Geometry check sheet. Reference: the model listing, model coordinates, mm. Face numbers are marked on the shaded views. A direction names the side the tool comes from. Give positions to 0.01 mm unless a question says otherwise; leave off trailing zeros. Loops run counter-clockwise (first coordinate to the right, second up) from the corner with the lowest first, then second, coordinate; pieces in that order, holes last.
```python
from build123d import *

# Parameters (mm, degrees)
SIDE_BASE_DEPTH                    = 0.5
SIDE_BASE_2_COUNT                  = 2
SIDE_BASE_2_PITCH                  = 50
FRONT_BACK_WALLS_REACH             = 60.566
BASE_SKETCH_W                      = 50.5
BASE_SKETCH_H                      = 13.2
BASE_SKETCH_W_2                    = 15.8
BASE_SKETCH_H_2                    = 11.998021326
BASE_DEPTH                         = 0.5
ATTACHMENT_BASE_SKETCH_W           = 16.8
ATTACHMENT_BASE_SKETCH_H           = 13.2
ATTACHMENT_BASE_SKETCH_W_2         = 15.8
ATTACHMENT_BASE_SKETCH_H_2         = 11.998021326
ATTACHMENT_BASE_DEPTH              = 7
PIPE_TOP_EXTRA_CUTAWAY_REACH       = 64.84
SKETCH11_W                         = 15.8
SKETCH11_H                         = 0.195081796
SKETCH1_W                          = 15.8
SKETCH1_H                          = 12.193103122
FAN_BASE_DEPTH                     = 0.1
LEFT_RIGHT_WALL_REMOVAL_DEPTH      = 59.566323483
LEFT_RIGHT_WALL_REMOVAL_DEPTH_BACK = 59.566323483
SKETCH6_W                          = 28.631700026
SKETCH6_H                          = 16.366666667
CUTAWAY_LEFT_DEPTH                 = 53.811785181
LEFT_WALL_DEPTH                    = 0.520740187
SKETCH9_W                          = 43.808738797
SKETCH9_H                          = 16.366666667
CUTAWAY_RIGHT_DEPTH                = 46.956653807
RIGHT_WALL_DEPTH                   = 0.781709206


with BuildPart() as part:
    # Side base sketch → Side base (new body)
    with BuildSketch(Plane.ZY):
        Polygon((0, 13.2), (8.491348573, 5), (19.491348573, 0.8030407), (27.491348573, -0.530292633), (19, -3.166666667), (6, -1), (0, 0), align=None)
    extrude(amount=-SIDE_BASE_DEPTH)


with BuildPart() as side_base_2_1:
    # Side base 2: pattern copy
    add(part.part.moved(Location(Vector(1, 0, 0) * (1 * SIDE_BASE_2_PITCH))))

    # Wall base sketch → Front back walls (add, up to next)
    with BuildSketch(Plane(origin=(0.5, 0, 0), x_dir=(0, 0, -1), z_dir=(1, 0, 0)), mode=Mode.PRIVATE) as front_back_walls_sk1:
        Polygon((0, 12.504918204), (-8.217574488, 4.569298766), (-19.359827502, 0.318064001), (-26.428993119, -0.860130268), (-27.491348573, -0.530292633), (-19.491348573, 0.8030407), (-8.491348573, 5), (0, 13.2), align=None)
    front_back_walls_tool1 = extrude(front_back_walls_sk1.sketch, amount=FRONT_BACK_WALLS_REACH, mode=Mode.PRIVATE) - side_base_2_1.part
    # Wall base sketch → Front back walls (add, up to next)
    with BuildSketch(Plane(origin=(0.5, 0, 0), x_dir=(0, 0, -1), z_dir=(1, 0, 0)), mode=Mode.PRIVATE) as front_back_walls_sk2:
        Polygon((0, 0.506896878), (-19, -2.659769789), (-19, -3.166666667), (0, 0), align=None)
    front_back_walls_tool2 = extrude(front_back_walls_sk2.sketch, amount=FRONT_BACK_WALLS_REACH, mode=Mode.PRIVATE) - side_base_2_1.part

    add(part.part)  # Front back walls merges part
    add(front_back_walls_tool1.solids().sort_by_distance((0.5, 8.759227, 4.323285))[0])
    add(front_back_walls_tool2.solids().sort_by_distance((0.5, -1.329885, 9.5))[0])

    # Base sketch → Base (add)
    with BuildSketch(Plane(origin=(0, 0, 0), x_dir=(-1, 0, 0), z_dir=(0, 0, -1))):
        with Locations((-25.25, 6.6)):
            Rectangle(BASE_SKETCH_W, BASE_SKETCH_H)
        with Locations((-42.1, 6.505907541)):
            Rectangle(BASE_SKETCH_W_2, BASE_SKETCH_H_2, mode=Mode.SUBTRACT)
    extrude(amount=BASE_DEPTH)

    # Attachment base sketch → Attachment base (add)
    with BuildSketch(Plane(origin=(0, 0, -0.5), x_dir=(-1, 0, 0), z_dir=(0, 0, -1))):
        with Locations((-42.1, 6.6)):
            Rectangle(ATTACHMENT_BASE_SKETCH_W, ATTACHMENT_BASE_SKETCH_H)
        with Locations((-42.1, 6.505907541)):
            Rectangle(ATTACHMENT_BASE_SKETCH_W_2, ATTACHMENT_BASE_SKETCH_H_2, mode=Mode.SUBTRACT)
    extrude(amount=ATTACHMENT_BASE_DEPTH)

    # Pipe top extra cutaway: up to this plane
    pipe_top_extra_cutaway_end = Plane(origin=(500000, 12.504918204, 0), z_dir=(0, 0.7193398003386524, 0.694658370458996))
    # Sketch11 → Pipe top extra cutaway (cut, up to the surface)
    with BuildSketch(Plane(origin=(0, 0, -7.5), x_dir=(-1, 0, 0), z_dir=(0, 0, -1)), mode=Mode.PRIVATE) as pipe_top_extra_cutaway_sk1:
        with Locations((-42.1, 12.602459102)):
            Rectangle(SKETCH11_W, SKETCH11_H)
    pipe_top_extra_cutaway_tool1 = split(extrude(pipe_top_extra_cutaway_sk1.sketch, amount=-PIPE_TOP_EXTRA_CUTAWAY_REACH, mode=Mode.PRIVATE), bisect_by=pipe_top_extra_cutaway_end, keep=Keep.BOTH, mode=Mode.PRIVATE)
    add(pipe_top_extra_cutaway_tool1.solids().sort_by_distance((42.1, 12.602459, -7.5))[0], mode=Mode.SUBTRACT)

    # Sketch4 → Left right wall removal (cut, two sides: drawn at the far end of the back side and taken through both)
    with BuildSketch(Plane(origin=(0.5, 0, 0), x_dir=(0, 0, -1), z_dir=(1, 0, 0)).offset(-LEFT_RIGHT_WALL_REMOVAL_DEPTH_BACK)):
        Polygon((-26.428993119, -0.860130268), (-19, -3.166666667), (-19, -2.659769789), (0, 0.506896878), (0, 12.504918204), (-8.217574488, 4.569298766), (-19.359827502, 0.318064001), align=None)
    extrude(amount=LEFT_RIGHT_WALL_REMOVAL_DEPTH + LEFT_RIGHT_WALL_REMOVAL_DEPTH_BACK, mode=Mode.SUBTRACT)

    # Sketch6 → Cutaway left (cut, through all)
    with BuildSketch(Plane(origin=(46.557451165, 0, 13.548248036), x_dir=(0.27941058312270783, 0, -0.9601717169543313), z_dir=(0.9601717169543312, 0, 0.2794105831227078))):
        with Locations((-0.205615565, 5.016666667)):
            Rectangle(SKETCH6_W, SKETCH6_H)
    extrude(amount=CUTAWAY_LEFT_DEPTH, mode=Mode.SUBTRACT)

    # Sketch7 → Left wall (add, along a direction that is not the sketch's normal)
    with BuildSketch(Plane(origin=(46.557451165, 0, 13.548248036), x_dir=(0.27941058312270806, 0, -0.9601717169543312), z_dir=(0.9601717169543312, 0, 0.27941058312270806))):
        Polygon((-5.67789268, -2.659769789), (-5.677892681, -3.166666667), (-13.415043221, -0.860130268), (-6.052645962, 0.318064001), (5.551791887, 4.569298766), (14.110234448, 12.504918204), (14.110234448, 0.506896878), align=None)
    extrude(amount=-LEFT_WALL_DEPTH, dir=(1, 0, 0))

    # Sketch9 → Cutaway right (cut, through all)
    with BuildSketch(Plane(origin=(13.512268511, 0, 16.268006796), x_dir=(0.7692529145051232, 0, -0.63894440566091), z_dir=(0.63894440566091, 0, 0.7692529145051232))):
        with Locations((4.338926024, 5.016666667)):
            Rectangle(SKETCH9_W, SKETCH9_H)
    extrude(amount=-CUTAWAY_RIGHT_DEPTH, mode=Mode.SUBTRACT)

    # Sketch10 → Right wall (add, along a direction that is not the sketch's normal)
    with BuildSketch(Plane(origin=(13.512268511, 0, 16.268006796), x_dir=(-0.7692529145051233, -2.5697854420108344e-15, 0.63894440566091), z_dir=(-0.6389444056609099, 0, -0.7692529145051232))):
        Polygon((-25.460754726, 12.504918204), (-25.460754725, 0.506896878), (4.275791728, -2.659769789), (4.275791728, -3.166666667), (15.902770622, -0.860130268), (4.838951055, 0.318064001), (-12.599581805, 4.569298766), align=None)
    extrude(amount=-RIGHT_WALL_DEPTH, dir=(-1, 0, 0))


with BuildPart() as body_2:
    # Sketch1 → Fan base (new body)
    with BuildSketch(Plane(origin=(0, 0, -7.5), x_dir=(-1, 0, 0), z_dir=(0, 0, -1))):
        with Locations((-42.1, 6.603448439)):
            Rectangle(SKETCH1_W, SKETCH1_H)
    extrude(amount=FAN_BASE_DEPTH)


solid = side_base_2_1.part
```
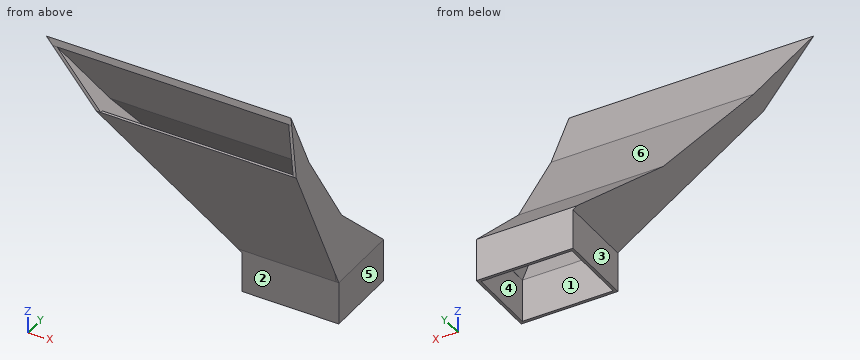
1) Sectioned sample at D-D on x = 15. Enter the section's corners in (y, z).
2) Tool access check on the marked faces 1, 2 and 3. Record the directions out of +Z, -Z, +X, -X, +Y, -Y that give a thin tool (end or side, any length) a straight path to the whole face; none if there is none.
3) Mould release check, pull along X, two halves, no side actions. Record for the marked faces 4, 5 and 6: +X half, -X half, draft (parallel to the pull), parting line (faces both ways), or undercut.
4) Sectioned sample at A-A on z = -4.5. Enter the section's corners in (x, y), plus the area to 3 significant figures.
5) Depth check by flat-ended pin: P1, Ø5.5, axis at y = 4, z = -2.5, coming from the -X side; P2, Ø3, axis at x = 38.5, y = 4, coming from the -Z side; P3, Ø8, axis at x = 41.5, z = -5.5, coming from the -Y side. Enter the tip coordinate at first touch or a pass-through.
6) Scan lines: line 1 along Y through (x, z) = (42, -1); line 2 along X through (y, z) = (9.75, -6); line 3 along X through (y, z) = (-0.5, 11). Record each from-to range of solid material in increasing order.
7) Sectioned sample at B-B on x = 35.5. Enter the section's corners in (y, z).
Determined:
1. outline: (-3.17, 19) - (-2.51, 15.03) - (2.5, 15.03) - (0.8, 19.49) - (-0.53, 27.49) - (-0.86, 26.43) - (0.32, 19.36) - (1.72, 15.68) - (-2.11, 15.68) - (-2.66, 19) - close
2. face 1: -Z
2. face 2: -Z, +X, -X, -Y
2. face 3: -Z, -X, +Y, -Y
3. face 4: undercut
3. face 5: +X half
3. face 6: draft
4. outline: (33.7, 0) - (50.5, 0) - (50.5, 13.2) - (33.7, 13.2) - close; hole (34.2, 0.51) - (50, 0.51) - (50, 12.7) - (34.2, 12.7) - close
4. area: 29.1 mm2
5. P1: stops at x = 32.8
5. P2: stops at z = 7.25
5. P3: stops at y = 0
6. line 1: y = 0 to 0.51, 12.7 to 13.2
6. line 2: x = 33.7 to 34.2, 50 to 50.5
6. line 3: x = 19.85 to 20.64, 46.78 to 47.3
7. outline: (-3.17, 19) - (0, 0) - (0, -7.5) - (0.51, -7.5) - (0.51, 0) - (-2.66, 19) - close; (-0.86, 26.43) - (0.32, 19.36) - (4.57, 8.22) - (12.7, -0.2) - (12.7, -7.5) - (13.2, -7.5) - (13.2, 0) - (5, 8.49) - (0.8, 19.49) - (-0.53, 27.49) - close
